from build123d import *

# Parameters (mm, degrees)
CROQUIS6_R              = 23.5
CORTAR_EXTRUIR2_DEPTH   = 0.5
CROQUIS7_R              = 3.05
CROQUIS7_R_2            = 1.55
SALIENTE_EXTRUIR1_DEPTH = 9.5
CORTAR_EXTRUIR3_START   = -5.5
CROQUIS8_R              = 1.55
CORTAR_EXTRUIR3_DEPTH   = 5.5
REDONDEO1_R             = 2
REDONDEO2_R             = 2
CROQUIS9_R              = 23.5
CORTAR_EXTRUIR4_DEPTH   = 1


with BuildPart() as part:
    # Croquis3 → Revolución1 (revolve)
    with BuildSketch(Plane.XY):
        with BuildLine():
            Line((25, 0), (25, 3.742571384))
            ThreePointArc((25, 3.742571384), (21.675655898, 5.498663982), (18.228756555, 7))
            ThreePointArc((18.228756555, 7), (16.801415582, 9.620779584), (15, 12))
            Line((15, 12), (0, 12))
            Line((0, 12), (0, 0))
            Line((0, 0), (25, 0))
        make_face()
    revolve(axis=Axis((0, 0, 0), (0, 1, 0)))

    # Croquis4 → Cortar-Revolución1 (revolve, cut)
    with BuildSketch(Plane.XY):
        with BuildLine():
            Line((0, 1.5), (0, 10.5))
            Line((0, 10.5), (14.30686093, 10.5))
            ThreePointArc((14.30686093, 10.5), (15.877398251, 8.266411941), (17.102065618, 5.825983099))
            ThreePointArc((17.102065618, 5.825983099), (20.35484662, 4.463230038), (23.5, 2.867708066))
            Line((23.5, 2.867708066), (23.5, 1.5))
            Line((23.5, 1.5), (0, 1.5))
        make_face()
    revolve(axis=Axis((0, 10.5, 0), (0, 1, 0)), mode=Mode.SUBTRACT)

    # Croquis6 → Cortar-Extruir2 (cut)
    with BuildSketch(Plane.XZ):
        with Locations(Location((0, 0, 0), (0, 0, 270))):
            Circle(CROQUIS6_R)
    extrude(amount=-CORTAR_EXTRUIR2_DEPTH, mode=Mode.SUBTRACT)

    # Croquis7 → Saliente-Extruir1 (add)
    # profile 1 of 2: a face of its own
    with BuildSketch(Plane.XZ.offset(-10.5)):
        with Locations(Location((0, 10, 0), (0, 0, 180))):
            Circle(CROQUIS7_R)
        with Locations((0, 10)):
            Circle(CROQUIS7_R_2, mode=Mode.SUBTRACT)
    # profile 2 of 2: a face of its own
    with BuildSketch(Plane.XZ.offset(-10.5)):
        with Locations(Location((0, -10, 0), (0, 0, 180))):
            Circle(CROQUIS7_R)
        with Locations(Location((0, -10, 0), (0, 0, 90))):
            Circle(CROQUIS7_R_2, mode=Mode.SUBTRACT)
    extrude(amount=SALIENTE_EXTRUIR1_DEPTH)

    # Croquis8 → Cortar-Extruir3 (cut)
    with BuildSketch(Plane.XZ.offset(-10.5).offset(CORTAR_EXTRUIR3_START)):
        with Locations((0, -10)):
            Circle(CROQUIS8_R)
        with Locations((0, 10)):
            Circle(CROQUIS8_R)
    extrude(amount=CORTAR_EXTRUIR3_DEPTH, mode=Mode.SUBTRACT)

    # Redondeo1
    redondeo1_edges = [part.edges().sort_by_distance(p)[0] for p in [
        (-15, 12, 0),
    ]]
    fillet(redondeo1_edges, radius=REDONDEO1_R)

    # Redondeo2
    redondeo2_edges = [part.edges().sort_by_distance(p)[0] for p in [
        (-25, 3.742571384, 0),
    ]]
    fillet(redondeo2_edges, radius=REDONDEO2_R)

    # Croquis9 → Cortar-Extruir4 (cut)
    with BuildSketch(Plane.XZ.offset(-0.5)):
        Circle(CROQUIS9_R)
    extrude(amount=-CORTAR_EXTRUIR4_DEPTH, mode=Mode.SUBTRACT)


solid = part.part
Check sheet for the modelled part. Datum: model origin and axes. Units: mm. A direction names the side the tool comes from. Round coordinates to 2 decimals unless told otherwise and drop trailing zeros. Write each loop counter-clockwise with the first axis right and the second up, starting at its lowest first coordinate (ties: lowest second). Pieces come first, ordered by that corner, then holes. Notation, with made-up numbers: (28.5, -24.5) -> (41.5, -24.5) arc R12 ccw to (41.5, -13.5) -> close; hole circle Ø11 at (71.25, -6.5). An arc over 180 degrees is marked (long way). Answer as CSV lines item,"result". Start each with the question number.
1) Section check A-A on y = 9. Enter the section's corners in (x, z), and give its area (3 significant figures).
2) Section check B-B on x = 0. State how many separate pieces and enclosed holes the cut face has, and give its area (3 significant figures).
3) Go/stop test with flat-tipped pins: P1, Ø2, axis at y = 3, z = 9, coming from the -X side; P2, Ø14.5, axis at x = -5.5, z = -2, coming from the -Y side; P3, Ø2.5, axis at x = 0, z = -10, coming from the -Y side; P4, Ø1.5, axis at x = -19.5, y = 3.5, coming from the +Z side. Record where each tip stops, or that it passes through.
4) Release check for a two-part mould opening along Z. For faces 1 (the flat face through (0, 12, 0)), 2 (the cylindrical face through (1.219, 6.823, -10.957)), 3 (the cylindrical face through (-1.64, 6.06, -12.57)), 4 (the cylindrical face through (23.846, 1.304, -7.509)) record: pulls with the +Z half, pulls with the -Z half, needs draft (parallel to the pull), parting line crosses it, or undercut.
5) Tool access check on faces 5 (the cylindrical face through (-0.336, 6.823, 8.487)), 6 (the cylindrical face through (-1.64, 6.06, 7.43)). Record the directions out of +Z, -Z, +X, -X, +Y, -Y that give a thin tool (end or side, any length) a straight path to the whole face; none if there is none.
6) Material ranges on line 1 (Z direction, x = 0, y = 1.15); line 2 (X direction, y = 8.75, z = 11), recorded low to high. Write a range as from..to.
Found:
1,outline,"circle Ø34.37 at (0, 0); circle Ø6.1 at (0, -10); circle Ø6.1 at (0, 10); hole circle Ø30.83 at (0, 0); hole circle Ø3.1 at (0, -10); hole circle Ø3.1 at (0, 10)"
1,area,"225 mm^2"
2,separate pieces,"3"
2,enclosed holes,"0"
2,area,"137 mm^2"
3,P1,"stops at x = -23.67"
3,P2,"stops at y = 1.5"
3,P3,"passes through"
3,P4,"stops at z = 16.31"
4,face 1,"needs draft"
4,face 2,"undercut"
4,face 3,"undercut"
4,face 4,"parting line crosses it"
5,face 5,"+Y, -Y"
5,face 6,"-Y"
6,line 1,"z = -25..-23.5, 23.5..25"
6,line 2,"x = -13.39..-11.03, -2.88..-1.18, 1.18..2.88, 11.03..13.39"
